Verification items for the finished model (mm, model axes). Coordinates: 2 decimals unless noted, no trailing zeros. Write each loop counter-clockwise with the first axis right and the second up, starting at its lowest first coordinate (ties: lowest second). Pieces come first, ordered by that corner, then holes. Notation, with made-up numbers: (37, 17) -> (82, 17) arc R26 cw to (82, 45) -> close; hole circle Ø4 at (72, 46.25). An arc over 180 degrees is marked (long way). Use CSV: the item, a comma, the result in double quotes.
Autodesk Inventor part; units mm, degrees
ref_plane "YZ Plane" through (0, 0, 0) normal (1, 0, 0) x (0, 1, 0)
ref_plane "XZ Plane" through (0, 0, 0) normal (0, 1, 0) x (-1, 0, 0)
ref_plane "XY Plane" through (0, 0, 0) normal (0, 0, 1) x (1, 0, 0)
sketch "Sketch1" plane through (0, 0, 0) normal (0, 0, 1) x (1, 0, 0)
  circle A0 centre (30, 0) radius 2.3
  circle A1 centre (30, 0) radius 6
  line L0 (24, 0) -> (24, 82.5)
  line L1 (36, 0) -> (36, 82.5)
  line L2 (24, 41.25) -> (36, 41.25) construction
  circle A2 centre (30, 82.5) radius 2.3
  circle A3 centre (30, 82.5) radius 6
  point P0 (0, 0)
  dimension "d0" = 12
  dimension "d1" = 82.5
extrude "Extrusion1" add sketch "Sketch1" along normal blind 3.2
properties part number "Eslabon_TransPot"
1) Mould release check, pull along Y, two halves, no side actions. Record for faces 1 (the flat face through (24, 41, 2)), 2 (the cylindrical face through (27.702, -0.101, 1.578)), 3 (the cylindrical face through (30, -6, 2)): released by +Y, released by -Y, zero draft, split by the parting line, or undercut.
Return value:
face 1,"zero draft"
face 2,"undercut"
face 3,"released by -Y"
2) Cross-section at B-B (y = 83.5). Record the boundary of the cut face in (x, z), plus the area to 3 significant figures.
Return value:
outline,"(24.08, 0) -> (27.93, 0) -> (27.93, 3.2) -> (24.08, 3.2) -> close; (32.07, 0) -> (35.92, 0) -> (35.92, 3.2) -> (32.07, 3.2) -> close"
area,"24.6 mm2"
3) Scan lines: L1, parallel to Y at x = 30, z = 2.55; L2, parallel to Y at x = 31.75, z = 2.3; L3, parallel to X at y = 81, z = 2.25. Record each from-to range of solid material in increasing order.
Return value:
L1,"-6 to -2.3, 2.3 to 80.2, 84.8 to 88.5"
L2,"-5.74 to -1.49, 1.49 to 81.01, 83.99 to 88.24"
L3,"24 to 28.26, 31.74 to 36"
4) Gauge pin test, flat end, axial feed: pin 1 (1.5 mm diameter, centred on x = 32, z = 2, fed in from -Y). Record the tip position at first contact, or that the pin passes through.
Return value:
pin 1,"y = -5.87"
5) Cross-section at C-C (z = 2.55). Record the boundary of the cut face in (x, y).
Return value:
outline,"(24, 0) arc R6 ccw to (36, 0) -> (36, 82.5) arc R6 ccw to (24, 82.5) -> close; hole circle Ø4.6 at (30, 0); hole circle Ø4.6 at (30, 82.5)"
6) Cross-section at A-A (x = 29). Record the boundary of the cut face in (y, z), plus the area to 3 significant figures.
Return value:
outline,"(-5.92, 0) -> (-2.07, 0) -> (-2.07, 3.2) -> (-5.92, 3.2) -> close; (2.07, 0) -> (80.43, 0) -> (80.43, 3.2) -> (2.07, 3.2) -> close; (84.57, 0) -> (88.42, 0) -> (88.42, 3.2) -> (84.57, 3.2) -> close"
area,"275 mm2"
